```python
from build123d import *

# Parameters (mm, degrees)
SKETCH011_W          = 95
SKETCH011_H          = 6.35
SKETCH011_R          = 1.6
PAD005_DEPTH         = 2.25
SKETCH012_W          = 30
SKETCH012_H          = 3
POCKET003_DEPTH      = 0.001
POCKET003_DEPTH_BACK = 2.251
PAD006_DEPTH         = 2.25
FILLET002_R          = 0.5
FILLET004_R          = 0.2
FILLET003_R          = 1
FILLET005_R          = 3


with BuildPart() as part:
    # Sketch011 → Pad005 (new body)
    with BuildSketch(Plane.XY):
        with Locations((0, 0.325)):
            Rectangle(SKETCH011_W, SKETCH011_H)
        with Locations((-42.5, 0)):
            Circle(SKETCH011_R, mode=Mode.SUBTRACT)
        with Locations((42.5, 0)):
            Circle(SKETCH011_R, mode=Mode.SUBTRACT)
        with Locations((-22.5, 0)):
            Circle(SKETCH011_R, mode=Mode.SUBTRACT)
        with Locations((22.5, 0)):
            Circle(SKETCH011_R, mode=Mode.SUBTRACT)
    extrude(amount=PAD005_DEPTH)

    # Sketch012 → Pocket003 (cut, two sides)
    with BuildSketch(Plane.XY) as pocket003_sk:
        with Locations((0, -1.35)):
            Rectangle(SKETCH012_W, SKETCH012_H)
    extrude(amount=-POCKET003_DEPTH, mode=Mode.SUBTRACT)
    extrude(pocket003_sk.sketch, amount=POCKET003_DEPTH_BACK, mode=Mode.SUBTRACT)

    # Sketch013 → Pad006 (join)
    with BuildSketch(Plane.XY):
        with BuildLine():
            ThreePointArc((-15, -1.85), (0, -4.423593), (15, -1.85))
            Line((15, -0.95), (15, -1.85))
            ThreePointArc((-15, -0.95), (0, -3.523593), (15, -0.95))
            Line((-15, -0.95), (-15, -1.85))
        make_face()
    extrude(amount=PAD006_DEPTH)

    # Fillet002
    fillet002_edges = [part.edges().sort_by_distance(p)[0] for p in [
        (15, 0.15, 1.125),
        (-15, 0.15, 1.125),
        (-15, -0.95, 1.125),
        (15, -0.95, 1.125),
        (-15, -1.85, 1.125),
        (15, -1.85, 1.125),
    ]]
    fillet(fillet002_edges, radius=FILLET002_R)

    # Fillet004
    fillet004_edges = [part.edges().sort_by_distance(p)[0] for p in [
        (15, -2.85, 1.125),
        (-15, -2.85, 1.125),
    ]]
    fillet(fillet004_edges, radius=FILLET004_R)

    # Fillet003
    fillet003_edges = [part.edges().sort_by_distance(p)[0] for p in [
        (-47.5, -2.85, 1.125),
        (47.5, -2.85, 1.125),
    ]]
    fillet(fillet003_edges, radius=FILLET003_R)

    # Fillet005
    fillet005_edges = [part.edges().sort_by_distance(p)[0] for p in [
        (-47.5, 3.5, 1.125),
        (47.5, 3.5, 1.125),
    ]]
    fillet(fillet005_edges, radius=FILLET005_R)


solid = part.part
```
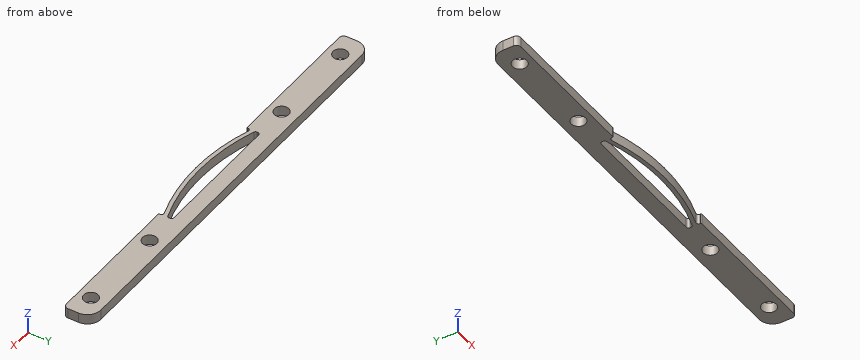
Verification items for the finished model (mm, model axes). Coordinates: 2 decimals unless noted, no trailing zeros. Write each loop counter-clockwise with the first axis right and the second up, starting at its lowest first coordinate (ties: lowest second). Pieces come first, ordered by that corner, then holes. Notation, with made-up numbers: M 19.5,-34 L 47.5,-34 A22 ccw 47.5,-21 Z; hole C 84,66 d3. An arc over 180 degrees is marked long. Answer as a JSON object with one key per item and string values. Group by question number.
(1) Material ranges on line 1 (Y direction, x = -42.5, z = 1.2); line 2 (X direction, y = -0.5, z = 2.1); line 3 (Y direction, x = 33, z = 1.4), recorded low to high.
(2) Cross-section at B-B, the plane x = -22.5. Record the cut outline in (y, z).
(3) Cross-section at C-C, the plane x = 2. Record the cut outline in (y, z), and give its area (3 significant figures).
(4) Gauge pin test, flat ends, axial feed: pin 1 (4 mm diameter, centred on x = 22.5, y = 0, fed in from +Z); pin 2 (0.7 mm diameter, centred on x = 29, z = 1, fed in from -Y); pin 3 (1 mm diameter, centred on x = -9, z = 0.5, fed in from -Y). Record the tip position at first contact, or that the pin passes through.
(5) Cross-section at A-A, the plane z = 0.7. Record the cut outline in (x, y).
Reply:
{
 "1": {"line 1": "-2.85 to -1.6, 1.6 to 3.5", "line 2": "-47.5 to -44.02, -40.98 to -24.02, -20.98 to -15, 15 to 20.98, 24.02 to 40.98, 44.02 to 47.5", "line 3": "-2.85 to 3.5"},
 "2": {"outline": "M -2.85,0 L -1.6,0 L -1.6,2.25 L -2.85,2.25 Z; M 1.6,0 L 3.5,0 L 3.5,2.25 L 1.6,2.25 Z"},
 "3": {"outline": "M -4.38,0 L -3.48,0 L -3.48,2.25 L -4.38,2.25 Z; M 0.15,0 L 3.5,0 L 3.5,2.25 L 0.15,2.25 Z", "area": "9.56 mm²"},
 "4": {"pin 1": "z = 2.25", "pin 2": "y = -2.85", "pin 3": "y = -3.61"},
 "5": {"outline": "M -47.5,-1.85 A1 ccw -46.5,-2.85 L -15.2,-2.85 A0.2 ccw -15,-2.65 L -15,-2.55 A0.5 cw -14.34,-2.08 A45 ccw 14.34,-2.08 A0.5 cw 15,-2.55 L 15,-2.65 A0.2 ccw 15.2,-2.85 L 46.5,-2.85 A1 ccw 47.5,-1.85 L 47.5,0.5 A3 ccw 44.5,3.5 L -44.5,3.5 A3 ccw -47.5,0.5 Z; hole C -42.5,0 d3.2; hole C -22.5,0 d3.2; hole M -15,-0.59 A0.5 ccw -14.66,-1.07 A45 ccw 14.66,-1.07 A0.5 ccw 15,-0.59 L 15,-0.35 A0.5 ccw 14.5,0.15 L -14.5,0.15 A0.5 ccw -15,-0.35 Z; hole C 22.5,0 d3.2; hole C 42.5,0 d3.2"}
}
